CAD build for the part. Positions are in the model's coordinates, mm. A direction names the side the tool comes from. Coordinates: 2 decimals unless noted, no trailing zeros. Order: outer loops, then holes, each group sorted by start corner. A loop starts at its lowest first (then second) coordinate and runs counter-clockwise, first axis right, second up. Notation, with made-up numbers: M -22.5,89.25 L 9.5,89.25 A23 ccw 9.5,100.25 Z; hole C -32,-12.75 d11. An arc over 180 degrees is marked long. Write item = value, one per line.
from build123d import *

# Parameters (mm, degrees)
F2_DEPTH = 3.175
F3_R     = 1.5875
F4_DEPTH = 25.4
F5_R     = 44.45
F6_DEPTH = 3.175
F6_TAPER = 10


# Not quite as in the source:
# - a feature of the source that left no trace in its solid (it failed there, or was rolled back) is left out


with BuildPart() as f2:
    # F1 (on Front) → F2 (new body)
    with BuildSketch(Plane.XZ):
        with BuildLine():
            Line((58.928, 65.278), (-58.928, 65.278))
            ThreePointArc((-58.928, 65.278), (-63.4181280605, 63.4181280605), (-65.278, 58.928))
            Line((-65.278, 58.928), (-65.278, -58.928))
            ThreePointArc((-65.278, -58.928), (-63.4181280605, -63.4181280605), (-58.928, -65.278))
            Line((-58.928, -65.278), (58.928, -65.278))
            ThreePointArc((58.928, -65.278), (63.4181280605, -63.4181280605), (65.278, -58.928))
            Line((65.278, -58.928), (65.278, 58.928))
            ThreePointArc((65.278, 58.928), (63.4181280605, 63.4181280605), (58.928, 65.278))
        make_face()
        with BuildLine():
            ThreePointArc((29.1683860123, 0), (21.2359008795, -15.4304684341), (4.5518055526, -20.1912078303))
            ThreePointArc((4.5518055526, -20.1912078303), (12.5076591177, -4.7892295638), (29.1683860123, 0))
        make_face(mode=Mode.SUBTRACT)
        with BuildLine():
            ThreePointArc((-30.0225467432, 26.633475086), (-11.3001914874, 17.269662026), (-5.1093608776, -2.7273676961))
            ThreePointArc((-5.1093608776, -2.7273676961), (-23.8921161087, 6.5851949341), (-30.0225467432, 26.633475086))
        make_face(mode=Mode.SUBTRACT)
        with BuildLine():
            Line((-5.3865113296, -11.8381703437), (-5.3865113296, -57.15))
            Line((-5.3865113296, -57.15), (-50.8, -57.15))
            ThreePointArc((-50.8, -57.15), (-55.2901280605, -55.2901280605), (-57.15, -50.8))
            Line((-57.15, -50.8), (-57.15, 50.8))
            ThreePointArc((-57.15, 50.8), (-55.2901280605, 55.2901280605), (-50.8, 57.15))
            Line((-50.8, 57.15), (50.8, 57.15))
            ThreePointArc((50.8, 57.15), (55.2901280605, 55.2901280605), (57.15, 50.8))
            Line((57.15, 50.8), (57.15, -50.8))
            ThreePointArc((57.15, -50.8), (55.2901280605, -55.2901280605), (50.8, -57.15))
            Line((50.8, -57.15), (2.8426104691, -57.15))
            Line((2.8426104691, -57.15), (2.8426104691, -28.5558674872))
            ThreePointArc((2.8426104691, -28.5558674872), (29.0723668952, -19.260680993), (37.6052677218, 7.2268673576))
            ThreePointArc((37.6052677218, 7.2268673576), (18.8257654598, 7.524261984), (3.0884773301, -2.7273676961))
            ThreePointArc((3.0884773301, -2.7273676961), (-7.830876963, 25.422268659), (-36.6427004337, 34.4507321715))
            ThreePointArc((-36.6427004337, 34.4507321715), (-32.213387286, 3.7443986853), (-5.3865113296, -11.8381703437))
        make_face(mode=Mode.SUBTRACT)
    extrude(amount=F2_DEPTH)

    # F3 (on face) → F4 (join)
    with BuildSketch(Plane(origin=(0, 0, -65.278), x_dir=(1, 0, 0), z_dir=(0, 0, -1))):
        with Locations((0, 1.5875)):
            Circle(F3_R)
    extrude(amount=F4_DEPTH)

    # F5 (on face) → F6 (join)
    with BuildSketch(Plane(origin=(0, 0, -90.678), x_dir=(1, 0, 0), z_dir=(0, 0, -1))):
        with Locations((0, 1.5875)):
            Circle(F5_R)
    extrude(amount=-F6_DEPTH, taper=F6_TAPER)


solid = f2.part
(1) Pull direction X, two halves, no side cores. Call faces 1 (the face through (63.467, -1.565, 63.368)), 2 (the face through (55.24, -1.57, 55.34)), 3 (the face through (-1, -3.175, 15)), 4 (the face through (-32.463, -1.565, 4.118)): +X half, -X half, draft (parallel to the pull), parting line (faces both ways), or undercut.
Evaluation:
face_1 = +X half
face_2 = undercut
face_3 = draft
face_4 = undercut
(2) Slice it at D-D, the plane z = 2.5. Write the cut outline in (x, y) (3 decimals).
Evaluation:
outline = M -65.278,-3.175 L -57.15,-3.175 L -57.15,0 L -65.278,0 Z; M -31.334,-3.175 L -19.545,-3.175 L -19.545,0 L -31.334,0 Z; M -5.083,-3.175 L 3.106,-3.175 L 3.106,0 L -5.083,0 Z; M 8.644,-3.175 L 37.947,-3.175 L 37.947,0 L 8.644,0 Z; M 57.15,-3.175 L 65.278,-3.175 L 65.278,0 L 57.15,0 Z
(3) Slice it at A-A, the plane z = -40.5. Write the cut outline in (x, y) (3 decimals).
Evaluation:
outline = M -65.278,-3.175 L -57.15,-3.175 L -57.15,0 L -65.278,0 Z; M -5.387,-3.175 L 2.843,-3.175 L 2.843,0 L -5.387,0 Z; M 57.15,-3.175 L 65.278,-3.175 L 65.278,0 L 57.15,0 Z
(4) Slice it at B-B, the plane z = 40. Write the cut outline in (x, y) (3 decimals).
Evaluation:
outline = M -65.278,-3.175 L -57.15,-3.175 L -57.15,0 L -65.278,0 Z; M 57.15,-3.175 L 65.278,-3.175 L 65.278,0 L 57.15,0 Z
(5) Pin check, flat tips, straight feed: pin 1 Ø3 at (x, z) = (9, 4.5) entering from -Y (3 decimals); pin 2 Ø6 at (x, z) = (-24.5, -9) entering from +Y. Stop position of each tip, or through.
Evaluation:
pin_1 = -3.175
pin_2 = through
(6) Slice it at C-C, the plane x = 53. Write the cut outline in (y, z) (3 decimals).
Evaluation:
outline = M -3.175,-65.278 L 0,-65.278 L 0,-56.757 L -3.175,-56.757 Z; M -3.175,56.757 L 0,56.757 L 0,65.278 L -3.175,65.278 Z
(7) Tool access for faces 5 (the face through (-1, 0, 15)), 6 (the face through (-1, -2, -90.678)), 7 (the face through (-11.5, -1.6, 17.5)): list every direction of +Z, -Z, +X, -X, +Y, -Y with a clear straight run to the whole face (end or side of a thin tool).
Evaluation:
face_5 = +Z, +X, -X, +Y
face_6 = -Z, +X, -X, +Y, -Y
face_7 = +Y, -Y
(8) Wall check: line 1 (Y direction, x = 18, z = -63) (3 decimals); line 2 (Z direction, x = 11.5, y = -22). Give the ranges that are in metal, low to high. Write a range as from..to.
Evaluation:
line_1 = -3.175..0
line_2 = -90.68..-87.5
